Autodesk Fusion 360 part; units mm, degrees
sketch "Esquisse1" plane through (0, 0, 0) normal (0, 0, 1) x (1, 0, 0)
  line L0 (0, 40) -> (70, 40)
  line L1 (70, 40) -> (70, 20)
  line L2 (70, 20) -> (0, 20)
  line L3 (0, 20) -> (0, 40)
  dimension "d1" = 70
  dimension "d2" = 20
extrude "Extrusion1" add sketch "Esquisse1" along normal blind 4
sketch "Esquisse2" plane through (0, 0, 0) normal (0, 0, -1) x (1, 0, 0)
  line L0 (70, -20) -> (0, -20)
  line L1 (0, -20) -> (0, -40)
  line L2 (0, -40) -> (70, -40)
  line L3 (70, -40) -> (70, -20)
  line L4 (7.5, -23) -> (12.5, -23)
  line L5 (12.5, -23) -> (12.5, -25)
  line L6 (12.5, -25) -> (7.5, -25)
  line L7 (7.5, -25) -> (7.5, -23)
  line L8 (10, -23) -> (10, -25) construction
  line L9 (35, -20) -> (35, -40) construction
  line L10 (57.5, -23) -> (57.5, -25)
  line L11 (62.5, -23) -> (57.5, -23)
  line L12 (62.5, -25) -> (62.5, -23)
  line L13 (57.5, -25) -> (62.5, -25)
  line L14 (0, -30) -> (70, -30) construction
  line L15 (7.5, -37) -> (12.5, -37)
  line L16 (12.5, -37) -> (12.5, -35)
  line L17 (12.5, -35) -> (7.5, -35)
  line L18 (7.5, -35) -> (7.5, -37)
  line L19 (62.5, -37) -> (57.5, -37)
  line L20 (62.5, -35) -> (62.5, -37)
  line L21 (57.5, -35) -> (62.5, -35)
  line L22 (57.5, -37) -> (57.5, -35)
  dimension "d5" = 25
extrude "Extrusion2" cut sketch "Esquisse2" against normal blind 2 contours L4 L5 L6 L7 | L10 L11 L12 L13 | L15 L16 L17 L18 | L19 L20 L21 L22
sketch "Esquisse3" plane through (0, 0, 4) normal (0, 0, 1) x (-1, 0, 0)
  line L0 (0, -20) -> (-70, -20)
  line L1 (-70, -20) -> (-70, -40)
  line L2 (-70, -40) -> (0, -40)
  line L3 (0, -40) -> (0, -20)
  line L4 (-22.5, -37.5) -> (-47.5, -37.5)
  line L5 (-47.5, -37.5) -> (-47.5, -22.5)
  line L6 (-47.5, -22.5) -> (-22.5, -22.5)
  line L7 (-22.5, -22.5) -> (-22.5, -37.5)
  line L8 (0, -30) -> (-70, -30) construction
  line L9 (-35, -40) -> (-35, -20) construction
  dimension "d8" = 25
  dimension "d9" = 15
extrude "Extrusion3" cut sketch "Esquisse3" against normal blind 2 contours L4 L5 L6 L7
Could you check a few things on this model? Use its own coordinates, in mm. A direction names the side the tool comes from. Round coordinates to 2 decimals unless told otherwise and drop trailing zeros. Order: outer loops, then holes, each group sorted by start corner. A loop starts at its lowest first (then second) coordinate and runs counter-clockwise, first axis right, second up.
Q1. Imagine slicing it at C-C, the plane y = 32. List the corners of the cut face in (x, z) for me.
Geometry says:
outline: (0, 0) - (70, 0) - (70, 4) - (47.5, 4) - (47.5, 2) - (22.5, 2) - (22.5, 4) - (0, 4) - close
Q2. I'm going to push a flat-ended pin straight in: P1, Ø1, axis at x = 10.5, y = 36, coming from the -Z side. Where does the tip first touch, or does it pass through?
Geometry says:
P1: stops at z = 2
Q3. Please list where these lines run through material, in increasing order: probe 1 along Y at (x, z) = (12, 0.55); probe 2 along X at (y, z) = (24, 1.9); probe 3 along X at (y, z) = (25, 2.25).
Geometry says:
probe 1: y = 20 to 23, 25 to 35, 37 to 40
probe 2: x = 0 to 7.5, 12.5 to 57.5, 62.5 to 70
probe 3: x = 0 to 22.5, 47.5 to 70
Q4. Which directions (+Z, -Z, +X, -X, +Y, -Y) give clear straight access to the entire face, cutting with the end or side of a thin tool? Please do faces 3 (the face through (35, 40, 2)), 4 (the face through (60, 23, 1)), 5 (the face through (35, 37.5, 3)).
Geometry says:
face 3: +Z, -Z, +X, -X, +Y
face 4: -Z
face 5: +Z
Q5. Imagine slicing it at B-B, the plane x = 35. List the corners of the cut face in (y, z) for me, then the cut area to 3 significant figures.
Geometry says:
outline: (20, 0) - (40, 0) - (40, 4) - (37.5, 4) - (37.5, 2) - (22.5, 2) - (22.5, 4) - (20, 4) - close
area: 50.0 mm2
Q6. Imagine slicing it at D-D, the plane x = 59. List the corners of the cut face in (y, z) for me.
Geometry says:
outline: (20, 0) - (23, 0) - (23, 2) - (25, 2) - (25, 0) - (35, 0) - (35, 2) - (37, 2) - (37, 0) - (40, 0) - (40, 4) - (20, 4) - close
Q7. Imagine slicing it at A-A, the plane z = 1.3. List the corners of the cut face in (x, y) for me, then the cut area to 3 significant figures.
Geometry says:
outline: (0, 20) - (70, 20) - (70, 40) - (0, 40) - close; hole (7.5, 23) - (12.5, 23) - (12.5, 25) - (7.5, 25) - close; hole (7.5, 35) - (12.5, 35) - (12.5, 37) - (7.5, 37) - close; hole (57.5, 23) - (62.5, 23) - (62.5, 25) - (57.5, 25) - close; hole (57.5, 35) - (62.5, 35) - (62.5, 37) - (57.5, 37) - close
area: 1,360 mm2
Q8. Thinking about a two-plate mould opening in X: for faces 1 (the face through (62.5, 24, 1)), 2 (the face through (35, 30, 0)), which applies, released by +X, released by -X, zero draft, split by the parting line, or undercut?
Geometry says:
face 1: undercut
face 2: zero draft
